Part model, mm, in its own coordinate system. Face numbers are marked on the shaded views. A direction names the side the tool comes from. Give positions to 0.01 mm unless a question says otherwise; leave off trailing zeros. Order: outer loops, then holes, each group sorted by start corner. A loop starts at its lowest first (then second) coordinate and runs counter-clockwise, first axis right, second up.
1. Slice it at C-C on z = 2.75. List the corners of the cut face in (x, y).
2. Drop flat-ended pins along their axis: pin 1 Ø3.5 at (x, y) = (0, 0.5) entering from +Z; pin 2 Ø4 at (x, z) = (-2.5, 3) entering from -Y; pin 3 Ø1.5 at (y, z) = (2.5, 6) entering from +X; pin 4 Ø1.5 at (x, y) = (-5.5, 0.5) entering from +Z. Give the stop position or say it passes through.
3. Slice it at A-A on y = 0. List the corners of the cut face in (x, z), and give its area (3 significant figures).
4. Probe line 1 (Z direction, x = -8.95, y = 0); line 2 (X direction, y = 2, z = 8.25); line 3 (Y direction, x = -1.7, z = 6.5). List the from-to ranges inside material, lowest first.
5. Which spindle directions (+Z, -Z, +X, -X, +Y, -Y) get a long thin tool onto all of the face, cutting with end or side? Do the marked faces 1 and 2. Say none if no direction does.
6. Mould opens along Y. For the marked faces 3, 4 and 5 say: +Y half, -Y half, draft (parallel to the pull), parting line (faces both ways), or undercut.
7. Slice it at B-B on x = 0. List the corners of the cut face in (y, z).
8. Slice it at D-D on x = -8. List the corners of the cut face in (y, z), and give its area (3 significant figures).
from build123d import *

# Parameters (mm, degrees)
CYLINDER001_R     = 2.5
CYLINDER001_DEPTH = 15
BOX_W             = 3
BOX_H             = 5.4
BOX_DEPTH         = 15
FILLET_R          = 1
BOX001_W          = 3
BOX001_H          = 6
BOX001_DEPTH      = 15
CYLINDER_R        = 10
CYLINDER_DEPTH    = 10


with BuildPart() as cilindro001:
    # Cylinder001 → Cylinder001 (new body)
    with BuildSketch(Plane(origin=(-15, 0, 6.5), x_dir=(0, 0, -1), z_dir=(1, 0, 0))):
        Circle(CYLINDER001_R)
    extrude(amount=CYLINDER001_DEPTH)


with BuildPart() as fillet_body:
    # Box → Box (new body)
    with BuildSketch(Plane(origin=(-1.5, -2.7, 0.6), x_dir=(1, 0, 0), z_dir=(0, 0, 1))):
        with Locations((1.5, 2.7)):
            Rectangle(BOX_W, BOX_H)
    extrude(amount=BOX_DEPTH)

    # Fillet
    fillet_edges = [fillet_body.edges().sort_by_distance(p)[0] for p in [
        (-1.5, -2.7, 8.1),
        (-1.5, 2.7, 8.1),
        (1.5, -2.7, 8.1),
        (1.5, 2.7, 8.1),
        (0, -2.7, 0.6),
        (0, -2.7, 15.6),
        (0, 2.7, 0.6),
        (0, 2.7, 15.6),
    ]]
    fillet(fillet_edges, radius=FILLET_R)


with BuildPart() as cubo001:
    # Box001 → Box001 (new body)
    with BuildSketch(Plane(origin=(-7, -3, 2.5), x_dir=(1, 0, 0), z_dir=(0, 0, 1))):
        with Locations((1.5, 3)):
            Rectangle(BOX001_W, BOX001_H)
    extrude(amount=BOX001_DEPTH)


with BuildPart() as cut002:
    # Cylinder → Cylinder (new body)
    with BuildSketch(Plane.XY):
        Circle(CYLINDER_R)
    extrude(amount=CYLINDER_DEPTH)

    # Cut: cut Cubo001
    add(cubo001.part, mode=Mode.SUBTRACT)

    # Cut001: cut Fillet body
    add(fillet_body.part, mode=Mode.SUBTRACT)

    # Cut002: cut Cilindro001
    add(cilindro001.part, mode=Mode.SUBTRACT)


solid = cut002.part
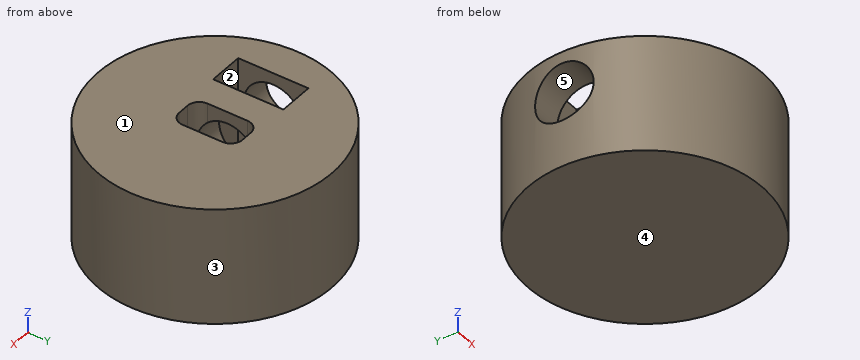
Data:
1. outline: circle Ø20 at (0, 0); hole (-7, -3) - (-4, -3) - (-4, 3) - (-7, 3) - close; hole (-1.5, -1.7) arc R1 ccw to (-0.5, -2.7) - (0.5, -2.7) arc R1 ccw to (1.5, -1.7) - (1.5, 1.7) arc R1 ccw to (0.5, 2.7) - (-0.5, 2.7) arc R1 ccw to (-1.5, 1.7) - close
2. pin 1: stops at z = 10
2. pin 2: stops at y = -9.99
2. pin 3: stops at x = 9.85
2. pin 4: stops at z = 2.5
3. outline: (-10, 0) - (10, 0) - (10, 10) - (1.5, 10) - (1.5, 0.6) - (-1.5, 0.6) - (-1.5, 4) - (-4, 4) - (-4, 2.5) - (-7, 2.5) - (-7, 4) - (-10, 4) - close; (-10, 9) - (-7, 9) - (-7, 10) - (-10, 10) - close; (-4, 9) - (-1.5, 9) - (-1.5, 10) - (-4, 10) - close
3. area: 122 mm2
4. line 1: z = 0 to 4, 9 to 10
4. line 2: x = -9.8 to -7, -4 to -1.45, 1.45 to 9.8
4. line 3: y = -9.85 to -2.5, 2.5 to 9.85
5. face 1: +Z, +X, -X, +Y, -Y
5. face 2: +Z
6. face 3: parting line
6. face 4: draft
6. face 5: undercut
7. outline: (-10, 0) - (10, 0) - (10, 10) - (2.7, 10) - (2.7, 1.6) arc R1 cw to (1.7, 0.6) - (-1.7, 0.6) arc R1 cw to (-2.7, 1.6) - (-2.7, 10) - (-10, 10) - close
8. outline: (-6, 0) - (6, 0) - (6, 10) - (-6, 10) - close; hole circle Ø5 at (0, 6.5)
8. area: 100 mm2
